```python
from build123d import *

# Parameters (mm, degrees)
F0_R     = 7.002224
F0_R_2   = 6.995584
F0_R_3   = 6.985
F1_DEPTH = 12.7
F2_R     = 5.08


with BuildPart() as f1:
    # F0 (on Front) → F1 (new body)
    with BuildSketch(Plane.XZ):
        with BuildLine():
            Line((37.680028, 111.202829), (-132.499972, 111.202829))
            ThreePointArc((-132.499972, 111.202829), (-146.868382, 105.251239), (-152.819972, 90.882829))
            Line((-152.819972, 90.882829), (-152.819972, -46.277171))
            ThreePointArc((-152.819972, -46.277171), (-150.588126, -51.665325), (-145.199972, -53.897171))
            Line((-145.199972, -53.897171), (-55.029972, -53.897171))
            Line((-55.029972, -53.897171), (-39.789972, -53.897171))
            Line((-39.789972, -53.897171), (50.380028, -53.897171))
            ThreePointArc((50.380028, -53.897171), (55.768182, -51.665325), (58.000028, -46.277171))
            Line((58.000028, -46.277171), (58.000028, 90.882829))
            ThreePointArc((58.000028, 90.882829), (52.048438, 105.251239), (37.680028, 111.202829))
        make_face()
        with Locations((-134.407488, -35.46943)):
            Circle(F0_R, mode=Mode.SUBTRACT)
        with Locations((-79.784476, -35.467136)):
            Circle(F0_R_2, mode=Mode.SUBTRACT)
        with Locations((-15.170232, -35.400602)):
            Circle(F0_R_3, mode=Mode.SUBTRACT)
        with Locations((39.581503, -35.505551)):
            Circle(F0_R_3, mode=Mode.SUBTRACT)
    extrude(amount=F1_DEPTH)

    # F2
    f2_edges = [f1.edges().sort_by_distance(p)[0] for p in [
        (52.048438, -12.7, 105.251239),
        (-47.409972, -12.7, 111.202829),
        (-146.868382, -12.7, 105.251239),
        (-152.819972, -12.7, 22.302829),
        (-150.588126, -12.7, -51.665325),
        (-47.409972, -12.7, -53.897171),
        (55.768182, -12.7, -51.665325),
        (58.000028, -12.7, 22.302829),
        (-141.409712, -12.7, -35.46943),
        (-86.78006, -12.7, -35.467136),
        (-22.155232, -12.7, -35.400602),
        (32.596503, -12.7, -35.505551),
    ]]
    fillet(f2_edges, radius=F2_R)


solid = f1.part
```
CAD build for the part. Positions are in the model's coordinates, mm. Give positions to 0.01 mm unless a question says otherwise; leave off trailing zeros. Order: outer loops, then holes, each group sorted by start corner. A loop starts at its lowest first (then second) coordinate and runs counter-clockwise, first axis right, second up.
(1) Drill centre lines: L1, parallel to X at y = -6.25, z = -37.5; L2, parallel to X at y = -7.5, z = -30.5; L3, parallel to Z at x = -14, y = -9.5. Where is each one in solid material? Low to high.
(2) Saw through at A-A, the plane y = -5. Give the cut face in (x, z) (1 decimal).
(3) Flat gauge pins, fed straight in: pin 1 (22.5 mm diameter, centred on x = -79.78, z = -35.47, fed in from -Y); pin 2 (1 mm diameter, centred on x = 1.5, y = -8.5, fed in from +Z). Where does each tip first touch, or does it go through?
Results found:
1. L1: x = -152.82 to -141.11, -127.71 to -86.48, -73.09 to -21.83, -8.51 to 32.89, 46.28 to 58
1. L2: x = -152.82 to -139.34, -129.47 to -84.71, -74.86 to -20.15, -10.19 to 34.71, 44.45 to 58
1. L3: z = -53.54 to -42.65, -28.15 to 110.84
2. outline: (-152.8, -46.3) arc R7.6 ccw to (-145.2, -53.9) - (50.4, -53.9) arc R7.6 ccw to (58, -46.3) - (58, 90.9) arc R20.3 ccw to (37.7, 111.2) - (-132.5, 111.2) arc R20.3 ccw to (-152.8, 90.9) - close; hole circle Ø14 at (-134.4, -35.5); hole circle Ø14 at (-79.8, -35.5); hole circle Ø14 at (-15.2, -35.4); hole circle Ø14 at (39.6, -35.5)
3. pin 1: stops at y = -12.63
3. pin 2: stops at z = 111.19
